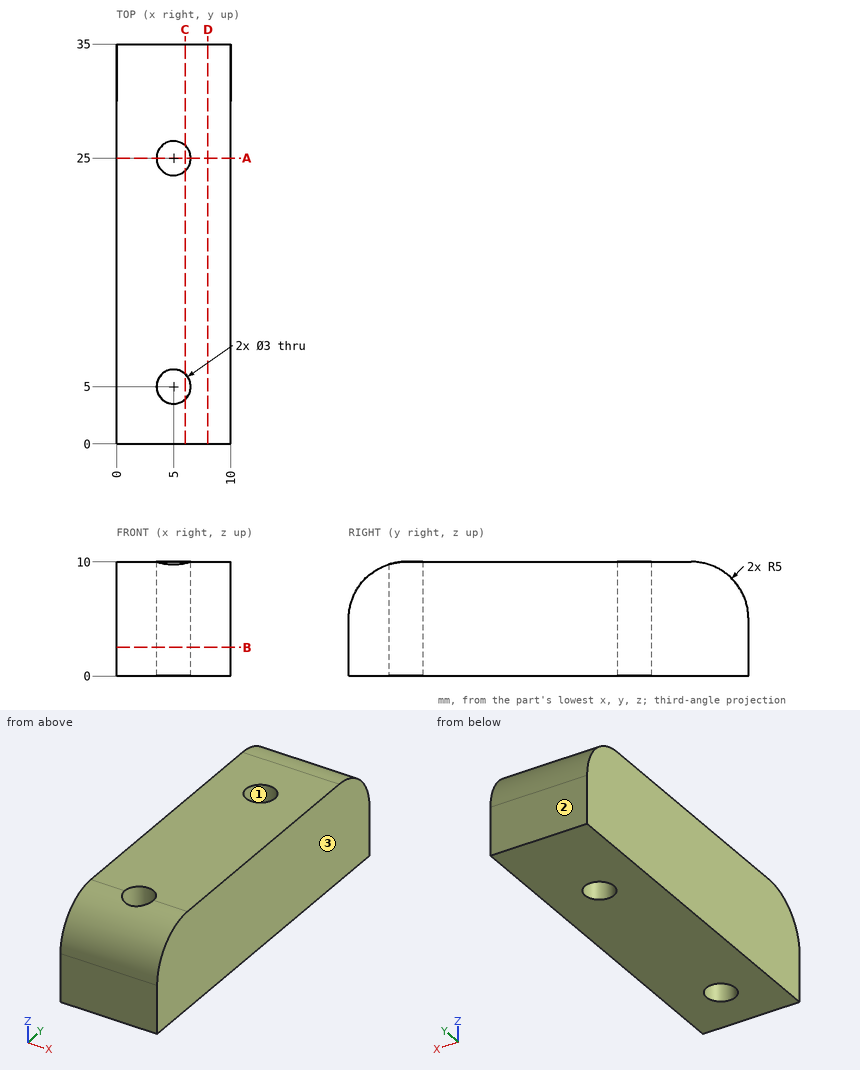
The figure shows three views and two pictorial views of one solid part (mm, origin at its lowest corner). Answer the questions. Give positions to 0.01 mm unless a question says otherwise; leave off trailing zeros. Loops run counter-clockwise (first coordinate to the right, second up) from the corner with the lowest first, then second, coordinate; pieces in that order, holes last. Notation, with made-up numbers: (51, 4.5) -> (84, 4.5) arc R37 cw to (84, 42.5) -> close; hole circle Ø10 at (50, -35). An arc over 180 degrees is marked (long way). Use a Markdown table: item, result. Add a question column.
1. Section C-C on x = 6 is taken. Determine the outline of the cut face in (y, z), and give its area (3 significant figures).
2. Section B-B on z = 2.5 is taken. Determine the outline of the cut face in (x, y), and give its area (3 significant figures).
3. Section D-D on x = 8 is taken. Determine the outline of the cut face in (y, z), and give its area (3 significant figures).
4. Determine the mould class of the marked faces 1, 2 and 3 for opening direction X: released by +X, released by -X, zero draft, split by the parting line, or undercut.
5. Find the intervals of material crossed by probe 1 along Y at (x, z) = (5, 4.75); probe 2 along Y at (x, z) = (5, 7.5); probe 3 along Y at (x, z) = (0.75, 7), in increasing order.
6. Flat-ended cylindrical pins translate along their axes: pin 1 Ø3 at (x, z) = (8.5, 7) entering from +Y; pin 2 Ø1.8 at (x, y) = (5, 25) entering from +Z. Find the tip coordinate at first contact, or state that the pin passes through.
7. Section A-A on y = 25 is taken. Determine the outline of the cut face in (x, z).
Results below:
| question | item | result |
|---|---|---|
| 1 | outline | (0, 0) -> (3.88, 0) -> (3.88, 9.87) arc R5 ccw to (0, 5) -> close; (6.12, 0) -> (23.88, 0) -> (23.88, 10) -> (6.12, 10) -> close; (26.12, 0) -> (35, 0) -> (35, 5) arc R5 ccw to (30, 10) -> (26.12, 10) -> close |
| 1 | area | 295 mm^2 |
| 2 | outline | (0, 0) -> (10, 0) -> (10, 35) -> (0, 35) -> close; hole circle Ø3 at (5, 5); hole circle Ø3 at (5, 25) |
| 2 | area | 336 mm^2 |
| 3 | outline | (0, 0) -> (35, 0) -> (35, 5) arc R5 ccw to (30, 10) -> (5, 10) arc R5 ccw to (0, 5) -> close |
| 3 | area | 339 mm^2 |
| 4 | face 1 | undercut |
| 4 | face 2 | zero draft |
| 4 | face 3 | released by +X |
| 5 | probe 1 | y = 0 to 3.5, 6.5 to 23.5, 26.5 to 35 |
| 5 | probe 2 | y = 0.67 to 3.5, 6.5 to 23.5, 26.5 to 34.33 |
| 5 | probe 3 | y = 0.42 to 34.58 |
| 6 | pin 1 | stops at y = 34.97 |
| 6 | pin 2 | passes through |
| 7 | outline | (0, 0) -> (3.5, 0) -> (3.5, 10) -> (0, 10) -> close; (6.5, 0) -> (10, 0) -> (10, 10) -> (6.5, 10) -> close |
